Solid Edge part; units mm, degrees
sketch "Sketch1" plane through (0, 0, 0) normal (1, 0, 0) x (0, 1, 0)
  line L0 (50, 59.6775) -> (117, 59.6775)
  line L1 (117, 59.6775) -> (117, 56.6775)
  line L2 (117, 56.6775) -> (50, 56.6775)
  line L3 (50, 59.6775) -> (50, 56.6775)
extrude "Protrusion1" add sketch "Sketch1" along normal mid plane 17
sketch "Sketch2" plane through (0, 84.5, 56.6775) normal (0, 0, -1) x (-1, 0, 0)
  line L0 (5, 28.5) -> (5, 32.5)
  line L1 (5, 32.5) -> (-5, 32.5)
  line L2 (-5, 32.5) -> (-5, 28.5)
  line L3 (-5, 28.5) -> (5, 28.5)
extrude "ExtrudedProtrusion_2" add sketch "Sketch2" along normal blind 7.5
fillet "Round_1" radius 3 1 edges at (0, 117, 49.1775)
fillet "Round_2" radius 2.5 2 edges at (-8.5, 50, 58.1775) (8.5, 50, 58.1775)
sketch "Sketch3" plane through (0, 84.5, 59.6775) normal (0, 0, 1) x (0, 1, 0)
  line L0 (-29.55, 0.95) -> (-21.45, 0.95)
  line L1 (-21.45, 0.95) -> (-21.45, 5.05)
  line L2 (-21.45, 5.05) -> (-29.55, 5.05)
  line L3 (-29.55, 5.05) -> (-29.55, 0.95)
extrude "Cutout1" cut sketch "Sketch3" against normal up to next
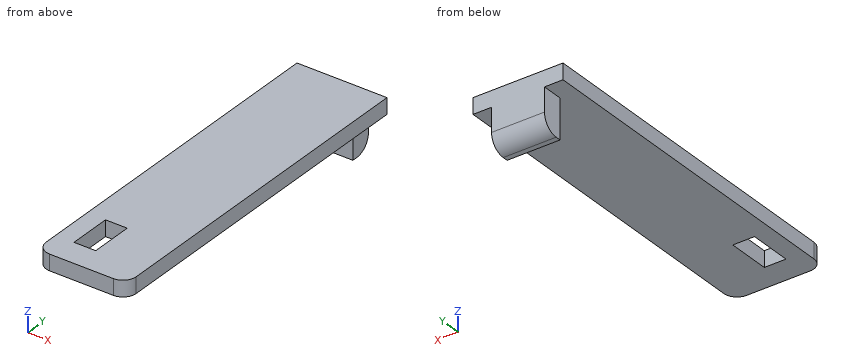
Here's how the part is built. I have some questions about the finished solid (model axes, mm). Give positions to 0.01 mm unless a question says otherwise; leave off trailing zeros. Order: outer loops, then holes, each group sorted by start corner. A loop starts at its lowest first (then second) coordinate and runs counter-clockwise, first axis right, second up. Notation, with made-up numbers: (-22.5, 24) -> (31.5, 24) arc R22 ccw to (31.5, 51) -> close; hole circle Ø5 at (22.25, 88.25). An arc over 180 degrees is marked (long way). One line per item, written item: value. Start each with the question number.
1. Imagine slicing it at C-C, the plane z = 57.25. List the corners of the cut face in (x, y) for me, plus the area to 3 significant figures.
2. Will these pins go through, and if not, where does the flat tip stop? pin 1 Ø5 at (x, y) = (-5.5, 65) entering from -Z; pin 2 Ø4.5 at (y, z) = (115.5, 52.5) entering from -X; pin 3 Ø1.2 at (y, z) = (114, 51.5) entering from +X.
3. Imagine slicing it at A-A, the plane y = 59.5. List the corners of the cut face in (x, z) for me.
4. Imagine slicing it at D-D, the plane x = 3. List the corners of the cut face in (y, z) for me.
5. Imagine slicing it at B-B, the plane x = -4. List the corners of the cut face in (y, z) for me, plus the area to 3 significant figures.
6. I need wall thicknesses on probe 1 along Y at (x, z) = (-3.5, 57.75); probe 2 along Z at (x, y) = (-5.5, 66.5); probe 3 along Y at (x, z) = (-4, 56.5). Which ranges of each line are inside material? Lowest first, please. Write a range as from..to.
Values follow:
1. outline: (-8.5, 52.5) arc R2.5 ccw to (-6, 50) -> (6, 50) arc R2.5 ccw to (8.5, 52.5) -> (8.5, 117) -> (-8.5, 117) -> close; hole (-5.05, 54.95) -> (-0.95, 54.95) -> (-0.95, 63.05) -> (-5.05, 63.05) -> close
1. area: 1,100 mm2
2. pin 1: stops at z = 56.68
2. pin 2: stops at x = -5
2. pin 3: stops at x = 5
3. outline: (-8.5, 56.68) -> (-5.05, 56.68) -> (-5.05, 59.68) -> (-8.5, 59.68) -> close; (-0.95, 56.68) -> (8.5, 56.68) -> (8.5, 59.68) -> (-0.95, 59.68) -> close
4. outline: (50, 56.68) -> (113, 56.68) -> (113, 49.18) -> (114, 49.18) arc R3 ccw to (117, 52.18) -> (117, 59.68) -> (50, 59.68) -> close
5. outline: (50, 56.68) -> (54.95, 56.68) -> (54.95, 59.68) -> (50, 59.68) -> close; (63.05, 56.68) -> (113, 56.68) -> (113, 49.18) -> (114, 49.18) arc R3 ccw to (117, 52.18) -> (117, 59.68) -> (63.05, 59.68) -> close
5. area: 205 mm2
6. probe 1: y = 50..54.95, 63.05..117
6. probe 2: z = 56.68..59.68
6. probe 3: y = 113..117
